The model under review builds one solid part; all positions refer to its coordinate system, in mm. Face numbers are marked on the shaded views. A direction names the side the tool comes from. Give positions to 0.01 mm unless a question says otherwise; leave off trailing zeros. Loops run counter-clockwise (first coordinate to the right, second up) from the corner with the lowest first, then second, coordinate; pieces in that order, holes last. Notation, with made-up numbers: (49, 5.5) -> (94, 5.5) arc R29 ccw to (94, 40.5) -> close; hole circle Ø9 at (45, 11.5). An arc over 180 degrees is marked (long way). Write each question's results on one line, items separated by ' | '. Start each with the question number.
Q1. Mouldability with a two-part tool opening along Y and no side actions: class the marked faces 6, 7 and 8 as released by +Y, released by -Y, zero draft, split by the parting line, or undercut.
Q2. Wall thickness on L1, parallel to Y at x = 15, z = -4.25; L2, parallel to Y at x = -21, z = 1; L3, parallel to X at y = 3.25, z = 0: over which ranges is each line inside the solid? List them lowest first. Write a range as [from, to].
Q3. We need section D-D (x = -11). Write out the cut boundary in (y, z) (3 decimals).
Q4. Machinability: for the marked faces 1, 2, 3, 4 and 5, which of the approach directions +Z, -Z, +X, -X, +Y, -Y give a long, thin tool a straight path to every point of the face, cutting with its end or side? Answer none if there is none.
Q5. We need section C-C (z = 0). Write out the cut boundary in (x, y), plus the area to 3 significant figures.
Q6. Insertion check: pin 1 Ø2.5 at (x, y) = (-3, 8) entering from -Z; pin 2 Ø1 at (y, z) = (-13.5, -6.5) entering from +X; pin 3 Ø2.5 at (x, y) = (5, 2) entering from -Z (3 decimals). Each pin has a flat end and moves straight along its axis. Give the tip position at first contact, or say it passes through.
Q7. We need section B-B (x = -20). Give the number of separate pieces and of enclosed holes in the cut face, plus the area to 3 significant figures.
Q8. We need section A-A (y = -9.5). Write out the cut boundary in (x, z).
from build123d import *

# Parameters (mm, degrees)
SKETCH001_W     = 18.4
SKETCH001_H     = 18.1
PAD001_DEPTH    = 28
SKETCH002_W     = 7.9
SKETCH002_H     = 47.6
POCKET_DEPTH    = 18.101
FILLET001_R     = 6.2
FILLET002_R     = 2
PAD_DEPTH       = 28
FILLET_R        = 2
SKETCH003_R     = 2.1
POCKET001_DEPTH = 10


with BuildPart() as socketbody:
    # Sketch001 → Pad001 (new body, symmetric)
    with BuildSketch(Plane.YZ):
        with Locations((-9.2, -2.1)):
            Rectangle(SKETCH001_W, SKETCH001_H)
    extrude(amount=PAD001_DEPTH, both=True)

    # Sketch002 (on Face1 of Pad001) → Pocket (cut, through all)
    with BuildSketch(Plane(origin=(0, 0, 6.95), x_dir=(0, -1, 0), z_dir=(0, 0, 1))):
        with Locations((10.25, 0)):
            Rectangle(SKETCH002_W, SKETCH002_H)
    extrude(amount=-POCKET_DEPTH, mode=Mode.SUBTRACT)

    # Fillet001
    fillet001_edges = [socketbody.edges().sort_by_distance(p)[0] for p in [
        (28, -18.4, -2.1),
        (-28, -18.4, -2.1),
    ]]
    fillet(fillet001_edges, radius=FILLET001_R)

    # Fillet002
    fillet002_edges = [socketbody.edges().sort_by_distance(p)[0] for p in [
        (-23.8, -10.25, 6.95),
        (0, -6.3, 6.95),
        (23.8, -10.25, 6.95),
        (0, -14.2, 6.95),
        (-23.8, -6.3, -2.1),
        (-28, -6.1, 6.95),
        (-26.184062, -16.584062, 6.95),
        (0, -18.4, 6.95),
        (26.184062, -16.584062, 6.95),
        (28, -6.1, 6.95),
        (0, 0, 6.95),
        (28, -6.1, -11.15),
        (26.184062, -16.584062, -11.15),
        (0, -18.4, -11.15),
        (-26.184062, -16.584062, -11.15),
        (28, 0, -2.1),
        (-28, 0, -2.1),
        (-28, -6.1, -11.15),
        (0, 0, -11.15),
        (0, -6.3, -11.15),
        (23.8, -10.25, -11.15),
        (0, -14.2, -11.15),
        (23.8, -14.2, -2.1),
        (-23.8, -10.25, -11.15),
        (-23.8, -14.2, -2.1),
        (23.8, -6.3, -2.1),
    ]]
    fillet(fillet002_edges, radius=FILLET002_R)


with BuildPart() as socketandrailbody:
    # Sketch → Pad (new body, symmetric)
    with BuildSketch(Plane.YZ):
        Polygon((-2, 4.125), (3.4, 4.125), (3.4, 6.95), (12.65, 6.95), (12.65, -6.95), (3.4, -6.95), (3.4, -4.125), (-2, -4.125), align=None)
    extrude(amount=PAD_DEPTH, both=True)

    # Fillet
    fillet_edges = [socketandrailbody.edges().sort_by_distance(p)[0] for p in [
        (-28, 8.025, 6.95),
        (0, 3.4, 6.95),
        (0, 12.65, 6.95),
        (28, 8.025, 6.95),
        (28, 12.65, 0),
        (0, 12.65, -6.95),
        (-28, 12.65, 0),
        (-28, 8.025, -6.95),
        (28, 8.025, -6.95),
        (0, 3.4, -6.95),
        (28, 3.4, -5.5375),
        (28, 3.4, 5.5375),
        (-28, 3.4, -5.5375),
        (-28, 0.7, -4.125),
        (28, 0.7, -4.125),
        (28, 0.7, 4.125),
        (-28, 0.7, 4.125),
        (-28, 3.4, 5.5375),
    ]]
    fillet(fillet_edges, radius=FILLET_R)

    # Sketch003 (on Face2 of Fillet) → Pocket001 (cut)
    with BuildSketch(Plane(origin=(0, -2, 0), x_dir=(0, 0, -1), z_dir=(0, -1, 0))):
        with Locations((0, 20)):
            Circle(SKETCH003_R)
        with Locations((0, -20)):
            Circle(SKETCH003_R)
    extrude(amount=-POCKET001_DEPTH, mode=Mode.SUBTRACT)

    # Fusion: union SocketBody
    add(socketbody.part)


solid = socketandrailbody.part
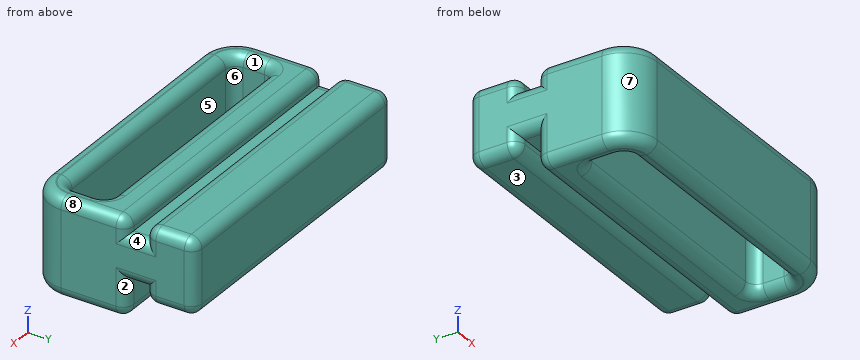
Output:
1) face 6: undercut | face 7: released by -Y | face 8: zero draft
2) L1: [-18.4, -14.2], [-6.3, 0], [3.4, 12.65] | L2: [-18.4, -14.2], [-6.3, 0], [8, 12.65] | L3: [-28, -22.1], [-17.9, 17.9], [22.1, 28]
3) outline: (-18.4, -9.15) arc R2 ccw to (-16.4, -11.15) -> (-16.2, -11.15) arc R2 ccw to (-14.2, -9.15) -> (-14.2, 4.95) arc R2 ccw to (-16.2, 6.95) -> (-16.4, 6.95) arc R2 ccw to (-18.4, 4.95) -> close; (-6.3, -9.15) arc R2 ccw to (-4.3, -11.15) -> (-2, -11.15) arc R2 ccw to (0, -9.15) -> (0, -4.125) -> (3.4, -4.125) -> (3.4, -4.95) arc R2 ccw to (5.4, -6.95) -> (10.65, -6.95) arc R2 ccw to (12.65, -4.95) -> (12.65, 4.95) arc R2 ccw to (10.65, 6.95) -> (5.4, 6.95) arc R2 ccw to (3.4, 4.95) -> (3.4, 4.125) -> (0, 4.125) -> (0, 4.95) arc R2 ccw to (-2, 6.95) -> (-4.3, 6.95) arc R2 ccw to (-6.3, 4.95) -> close
4) face 1: +Z | face 2: -Z, +X | face 3: -Z, +X, -X, +Y | face 4: +Z, +X | face 5: +Z, -Z
5) outline: (-28, -12.2) arc R6.2 ccw to (-21.8, -18.4) -> (21.8, -18.4) arc R6.2 ccw to (28, -12.2) -> (28, 10.65) arc R2 ccw to (26, 12.65) -> (-26, 12.65) arc R2 ccw to (-28, 10.65) -> close; hole (-23.8, -12.2) arc R2 ccw to (-21.8, -14.2) -> (21.8, -14.2) arc R2 ccw to (23.8, -12.2) -> (23.8, -8.3) arc R2 ccw to (21.8, -6.3) -> (-21.8, -6.3) arc R2 ccw to (-23.8, -8.3) -> close; hole (-22.1, 0) -> (-17.9, 0) -> (-17.9, 8) -> (-22.1, 8) -> close; hole (17.9, 0) -> (22.1, 0) -> (22.1, 8) -> (17.9, 8) -> close | area: 1,280 mm2
6) pin 1: z = -6.95 | pin 2: x = 27.95 | pin 3: z = -4.125
7) separate pieces: 2 | enclosed holes: 1 | area: 303 mm2
8) outline: (-28, -9.15) arc R2 ccw to (-26, -11.15) -> (-25.8, -11.15) arc R2 ccw to (-23.8, -9.15) -> (-23.8, 4.95) arc R2 ccw to (-25.8, 6.95) -> (-26, 6.95) arc R2 ccw to (-28, 4.95) -> close; (23.8, -9.15) arc R2 ccw to (25.8, -11.15) -> (26, -11.15) arc R2 ccw to (28, -9.15) -> (28, 4.95) arc R2 ccw to (26, 6.95) -> (25.8, 6.95) arc R2 ccw to (23.8, 4.95) -> close
